Input: part model. Units: mm. Frame: model coordinates. A direction names the side the tool comes from. Coordinates: 2 decimals unless noted, no trailing zeros. Write each loop counter-clockwise with the first axis right and the second up, starting at its lowest first coordinate (ties: lowest second). Pieces come first, ordered by that corner, then holes.
1) Set-up query: faces 3 (the flat face through (153, 0.25, -1)), 4 (the flat face through (153, 2.25, -1)), 5 (the cylindrical face through (-116.61, -0.99, -58.62)), 6 (the flat face through (-2, 0, 19)), 7 (the flat face through (-2, -2, 19)). Return all of +Z, -Z, +X, -X, +Y, -Y with unobstructed straight access to the full face (end or side cutting, diameter ignored); none if empty.
2) Draft query along Z for faces 1 (the flat face through (-153, 0.25, -1)), 2 (the cylindrical face through (-0.233, -0.986, -59.135)). Return one class per face: pulls with the +Z half, pulls with the -Z half, needs draft (parallel to the pull), parting line crosses it, or undercut.
3) Pin query (flat end, axial travel): pin 1 Ø2 at (y, z) = (-1, 93) entering from -X; pin 2 Ø9.5 at (x, z) = (-156.5, 22.5) entering from -Y; pin 3 Ø3 at (x, z) = (155, 75) entering from +Y; pin 4 Ø4 at (x, z) = (155, -75) entering from +Y. Return the tip coordinate at first contact, or that it passes through.
4) Section query C-C (x = -55). Output: boundary loops of the cut face in (y, z).
5) Section query D-D (z = 53.5). Output: boundary loops of the cut face in (x, y).
6) Section query B-B (z = -60.5). Output: boundary loops of the cut face in (x, y), then the cut area to 3 significant figures.
7) Line query: L1, parallel to Z at x = -155, y = 1.1; L2, parallel to X at y = 1, z = -75; L3, parallel to X at y = 1.5, z = -75. Output: solid intervals per line, ascending.
8) Section query A-A (x = 20.5). Output: boundary loops of the cut face in (y, z), then the cut area to 3 significant figures.
from build123d import *

# Parameters (mm, degrees)
SKETCH_1_W             = 320
SKETCH_1_H             = 182.5
SM_BASE_FLANGE_1_DEPTH = 2
OTHER_START            = -91.25
OTHER_1_DEPTH          = 182.5
OTHER_1_2_DEPTH        = 182.5
OTHER_4_DEPTH          = 182.5
OTHER_4_2_DEPTH        = 182.5
SKETCH_8_R             = 1.6
CUT_EXTRUDE_1_DEPTH    = 10
EXTRUDE_1_DEPTH        = 93.5
EXTRUDE_1_DEPTH_BACK   = 93.5
SKETCH_9_W             = 289.740046506
SKETCH_9_H             = 2
CUT_EXTRUDE_2_DEPTH    = 93.75


# Read off the part's stored shape, not the designer's step: Изгиб1, Изгиб4
# Sheet-metal steps are written as plain solids
with BuildPart() as part:
    # Sketch 1 → Базовая кромка1 (new body)
    with BuildSketch(Plane(origin=(0, 0, 0), x_dir=(1, 0, 0), z_dir=(0, 1, 0))):
        Rectangle(SKETCH_1_W, SKETCH_1_H)
    extrude(amount=-SM_BASE_FLANGE_1_DEPTH)

    # Other 1 outline → Other 1 (cut)
    with BuildSketch(Plane.XY.offset(OTHER_START)):
        with BuildLine():
            ThreePointArc((-144.820023253, -2), (-146.188323253, -1.63336512), (-147.189988373, -0.6317))
            Line((-147.189988373, -0.6317), (-147.486400002, -0.1183))
            ThreePointArc((-147.486400002, -0.1183), (-147.525930573, -0.05704621), (-147.571322452, 0))
            Line((-147.571322452, 0), (-160, 0))
            Line((-160, 0), (-160, -2))
            Line((-160, -2), (-144.820023253, -2))
        make_face()
    extrude(amount=OTHER_1_DEPTH, mode=Mode.SUBTRACT)

    # Other 1 2 outline → Other 1 2 (add)
    with BuildSketch(Plane.XY.offset(OTHER_START)):
        with BuildLine():
            ThreePointArc((-148.124314314, 0.25), (-147.820875688, 0.184596365), (-147.571322452, 0))
            Line((-147.571322452, 0), (-144.820023253, 0))
            ThreePointArc((-144.820023253, 0), (-145.188323253, 0.098685688), (-145.457937566, 0.3683))
            Line((-145.457937566, 0.3683), (-145.754349194, 0.8817))
            ThreePointArc((-145.754349194, 0.8817), (-146.756014314, 1.88336512), (-148.124314314, 2.25))
            Line((-148.124314314, 2.25), (-160, 2.25))
            Line((-160, 2.25), (-160, 0.25))
            Line((-160, 0.25), (-148.124314314, 0.25))
        make_face()
    extrude(amount=OTHER_1_2_DEPTH)

    # Other 4 outline → Other 4 (cut)
    with BuildSketch(Plane.XY.offset(OTHER_START)):
        with BuildLine():
            Line((160, 0), (147.671322452, 0))
            ThreePointArc((147.671322452, 0), (147.625930573, -0.05704621), (147.586400002, -0.1183))
            Line((147.586400002, -0.1183), (147.289988373, -0.6317))
            ThreePointArc((147.289988373, -0.6317), (146.288323253, -1.63336512), (144.920023253, -2))
            Line((144.920023253, -2), (160, -2))
            Line((160, -2), (160, 0))
        make_face()
    extrude(amount=OTHER_4_DEPTH, mode=Mode.SUBTRACT)

    # Other 4 2 outline → Other 4 2 (add)
    with BuildSketch(Plane.XY.offset(OTHER_START)):
        with BuildLine():
            Line((148.224314314, 0.25), (160, 0.25))
            Line((160, 0.25), (160, 2.25))
            Line((160, 2.25), (148.224314314, 2.25))
            ThreePointArc((148.224314314, 2.25), (146.856014314, 1.88336512), (145.854349194, 0.8817))
            Line((145.854349194, 0.8817), (145.557937566, 0.3683))
            ThreePointArc((145.557937566, 0.3683), (145.288323253, 0.098685688), (144.920023253, 0))
            Line((144.920023253, 0), (147.671322452, 0))
            ThreePointArc((147.671322452, 0), (147.920875688, 0.184596365), (148.224314314, 0.25))
        make_face()
    extrude(amount=OTHER_4_2_DEPTH)

    # Эскиз8 → Вырез-Вытянуть1 (cut)
    with BuildSketch(Plane(origin=(0, 2.25, 0), x_dir=(1, 0, 0), z_dir=(0, 1, 0))):
        with Locations(Location((-155, 0, 0), (0, 0, 270))):
            Circle(SKETCH_8_R)
        with Locations(Location((-155, 75, 0), (0, 0, 270))):
            Circle(SKETCH_8_R)
        with Locations(Location((-155, -75, 0), (0, 0, 270))):
            Circle(SKETCH_8_R)
        with Locations(Location((155, -75, 0), (0, 0, 270))):
            Circle(SKETCH_8_R)
        with Locations(Location((155, 75, 0), (0, 0, 270))):
            Circle(SKETCH_8_R)
        with Locations(Location((155, 0, 0), (0, 0, 270))):
            Circle(SKETCH_8_R)
    extrude(amount=-CUT_EXTRUDE_1_DEPTH, mode=Mode.SUBTRACT)

    # Эскиз9 → Бобышка-Вытянуть1 (add, two sides: drawn at the far end of the back side and taken through both)
    with BuildSketch(Plane.XY.offset(-EXTRUDE_1_DEPTH_BACK)):
        with Locations((0.05, -1)):
            Rectangle(SKETCH_9_W, SKETCH_9_H)
    extrude(amount=EXTRUDE_1_DEPTH + EXTRUDE_1_DEPTH_BACK)

    # Эскиз10 → Вырез-Вытянуть2 (cut)
    with BuildSketch(Plane(origin=(0, 0, 0), x_dir=(1, 0, 0), z_dir=(0, 1, 0))):
        with BuildLine():
            Line((-12.037112187, 47.06815468), (-104.806151311, 47.06815468))
            ThreePointArc((-104.806151311, 47.06815468), (-116.613119927, 58.875123295), (-104.806151311, 70.682091911))
            Line((-104.806151311, 70.682091911), (-12.037112187, 70.682091911))
            ThreePointArc((-12.037112187, 70.682091911), (-0.230143571, 58.875123295), (-12.037112187, 47.06815468))
        make_face()
        with BuildLine():
            Line((-32.558748115, 27.670991954), (94.506723655, 27.670991954))
            ThreePointArc((94.506723655, 27.670991954), (108.843756974, 13.333958635), (94.506723655, -1.003074685))
            Line((94.506723655, -1.003074685), (-32.558748115, -1.003074685))
            ThreePointArc((-32.558748115, -1.003074685), (-46.895781434, 13.333958635), (-32.558748115, 27.670991954))
        make_face()
        with BuildLine():
            Line((-89.244817746, -35.777942633), (-32.143884778, -35.777942633))
            ThreePointArc((-32.143884778, -35.777942633), (-21.089903693, -46.831923718), (-32.143884778, -57.885904803))
            Line((-32.143884778, -57.885904803), (-89.244817746, -57.885904803))
            ThreePointArc((-89.244817746, -57.885904803), (-100.298798831, -46.831923718), (-89.244817746, -35.777942633))
        make_face()
    extrude(amount=-CUT_EXTRUDE_2_DEPTH, mode=Mode.SUBTRACT)


solid = part.part
Answer:
1. face 3: +Z, -Z, +X, -Y
1. face 4: +Z, -Z, +X, -X, +Y
1. face 5: +Y, -Y
1. face 6: +Z, -Z, +Y
1. face 7: +Z, -Z, +X, -X, -Y
2. face 1: needs draft
2. face 2: undercut
3. pin 1: stops at x = -144.82
3. pin 2: stops at y = 0.25
3. pin 3: passes through
3. pin 4: stops at y = 2.25
4. outline: (-2, -93.5) - (0, -93.5) - (0, -70.68) - (-2, -70.68) - close; (-2, -47.07) - (0, -47.07) - (0, 35.78) - (-2, 35.78) - close; (-2, 57.89) - (0, 57.89) - (0, 93.5) - (-2, 93.5) - close
5. outline: (-160, 0.25) - (-148.12, 0.25) arc R0.74 cw to (-147.49, -0.12) - (-147.19, -0.63) arc R2.74 ccw to (-144.82, -2) - (-98.06, -2) - (-98.06, 0) - (-144.82, 0) arc R0.74 cw to (-145.46, 0.37) - (-145.75, 0.88) arc R2.74 ccw to (-148.12, 2.25) - (-160, 2.25) - close; (-23.33, -2) - (144.92, -2) arc R2.74 ccw to (147.29, -0.63) - (147.59, -0.12) arc R0.74 cw to (148.22, 0.25) - (160, 0.25) - (160, 2.25) - (148.22, 2.25) arc R2.74 ccw to (145.85, 0.88) - (145.56, 0.37) arc R0.74 cw to (144.92, 0) - (-23.33, 0) - close
6. outline: (-160, 0.25) - (-148.12, 0.25) arc R0.74 cw to (-147.49, -0.12) - (-147.19, -0.63) arc R2.74 ccw to (-144.82, -2) - (-116.5, -2) - (-116.5, 0) - (-144.82, 0) arc R0.74 cw to (-145.46, 0.37) - (-145.75, 0.88) arc R2.74 ccw to (-148.12, 2.25) - (-160, 2.25) - close; (-0.34, -2) - (144.92, -2) arc R2.74 ccw to (147.29, -0.63) - (147.59, -0.12) arc R0.74 cw to (148.22, 0.25) - (160, 0.25) - (160, 2.25) - (148.22, 2.25) arc R2.74 ccw to (145.85, 0.88) - (145.56, 0.37) arc R0.74 cw to (144.92, 0) - (-0.34, 0) - close
6. area: 411 mm2
7. L1: z = -91.25 to -76.6, -73.4 to -1.6, 1.6 to 73.4, 76.6 to 91.25
7. L2: x = -160 to -156.6, -153.4 to -145.83, 145.93 to 153.4, 156.6 to 160
7. L3: x = -160 to -156.6, -153.4 to -146.24, 146.34 to 153.4, 156.6 to 160
8. outline: (-2, -93.5) - (0, -93.5) - (0, -27.67) - (-2, -27.67) - close; (-2, 1) - (0, 1) - (0, 93.5) - (-2, 93.5) - close
8. area: 317 mm2
